Verification items for the finished model (mm, model axes). Face numbers are marked on the shaded views. A direction names the side the tool comes from. Coordinates: 2 decimals unless noted, no trailing zeros. Loops run counter-clockwise (first coordinate to the right, second up) from the corner with the lowest first, then second, coordinate; pieces in that order, holes last.
Q1. Sectioned sample at A-A (x = -2). Enter the section's corners in (y, z), then the cut area to 4 significant figures.
Q2. Sectioned sample at B-B (z = 20). Count the separate pieces of the cut face and the enclosed holes in it, then the cut area to 3 significant figures.
Q3. Mould release check, pull along X, two halves, no side actions. Record for the marked faces 1, 2, 3 and 4: +X half, -X half, draft (parallel to the pull), parting line (faces both ways), or undercut.
Q4. Sectioned sample at C-C (y = -6). Enter the section's corners in (x, z).
Q5. Material ranges on probe 1 along X at (y, z) = (-10, 34); probe 2 along Y at (x, z) = (-66.5, 18); probe 3 along Y at (x, z) = (83, 35), recorded low to high.
Q6. Access from +Z, -Z, +X, -X, +Y, -Y to the whole of each face (thin tool, end or side, straight path). Record for the marked faces 5 and 6.
Q7. Go/stop test with flat-tipped pins: P1, Ø1.2, axis at x = 27.5, z = 39.5, coming from the -Y side; P2, Ø0.8, axis at y = 28, z = 39, coming from the +X side; P3, Ø4, axis at x = 83, y = -35, coming from the +Z side. Record where each tip stops, or that it passes through.
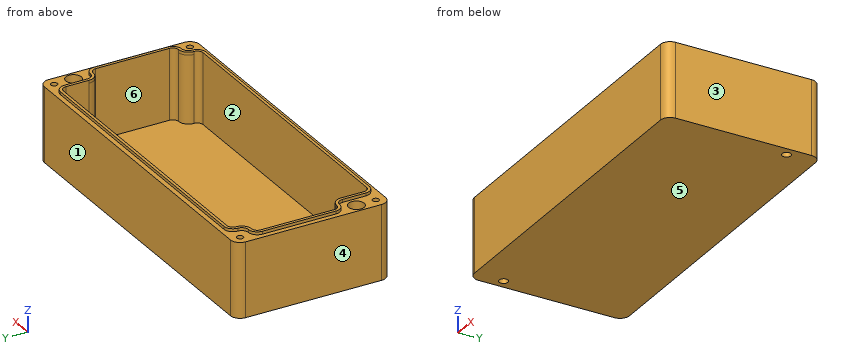
```python
from build123d import *

# Parameters (mm, degrees)
SKETCH1_W                                   = 176
SKETCH1_H                                   = 80
BOSS_EXTRUDE1_DEPTH                         = 38.5
SKETCH2_W                                   = 168
SKETCH2_H                                   = 72
CUT_EXTRUDE1_DEPTH                          = 35
FILLET2_R                                   = 5
SKETCH8_W                                   = 8
SKETCH8_H                                   = 20
SKETCH8_H_2                                 = 8
BOSS_EXTRUDE2_DEPTH                         = 35
FILLET4_R                                   = 3
FILLET5_R                                   = 5
M4_TAPPED_HOLE1_D                           = 3.3
M4_TAPPED_HOLE1_DEPTH                       = 11.5
M4_TAPPED_HOLE1_TIP                         = 0.991420021
BOSS_EXTRUDE3_START                         = 1.5
BOSS_EXTRUDE3_DEPTH                         = 1.5
CBORE_FOR_M4_CHEESE_HEAD_SCREW1_D           = 4.5
CBORE_FOR_M4_CHEESE_HEAD_SCREW1_CBORE_D     = 8
CBORE_FOR_M4_CHEESE_HEAD_SCREW1_CBORE_DEPTH = 30


with BuildPart() as part:
    # Sketch1 → Boss-Extrude1 (new body)
    with BuildSketch(Plane.XY):
        Rectangle(SKETCH1_W, SKETCH1_H)
    extrude(amount=BOSS_EXTRUDE1_DEPTH)

    # Sketch2 → Cut-Extrude1 (cut)
    with BuildSketch(Plane.XY.offset(38.5)):
        Rectangle(SKETCH2_W, SKETCH2_H)
    extrude(amount=-CUT_EXTRUDE1_DEPTH, mode=Mode.SUBTRACT)

    # Fillet2
    fillet2_edges = [part.edges().sort_by_distance(p)[0] for p in [
        (-88, 40, 19.25),
        (88, 40, 19.25),
        (88, -40, 19.25),
        (-88, -40, 19.25),
    ]]
    fillet(fillet2_edges, radius=FILLET2_R)

    # Sketch8 → Boss-Extrude2 (add)
    with BuildSketch(Plane.XY.offset(3.5)):
        with Locations((80, 26)):
            Rectangle(SKETCH8_W, SKETCH8_H)
        with Locations((80, -32)):
            Rectangle(SKETCH8_W, SKETCH8_H_2)
        with Locations((-80, -26)):
            Rectangle(SKETCH8_W, SKETCH8_H)
        with Locations((-80, 32)):
            Rectangle(SKETCH8_W, SKETCH8_H_2)
    extrude(amount=BOSS_EXTRUDE2_DEPTH)

    # Fillet4
    fillet4_edges = [part.edges().sort_by_distance(p)[0] for p in [
        (76, 36, 21),
        (84, 16, 21),
        (84, -28, 21),
        (76, -36, 21),
        (-76, -36, 21),
        (-84, -16, 21),
        (-84, 28, 21),
        (-76, 36, 21),
    ]]
    fillet(fillet4_edges, radius=FILLET4_R)

    # Fillet5
    fillet5_edges = [part.edges().sort_by_distance(p)[0] for p in [
        (-76, -16, 21),
        (76, -28, 21),
        (76, 16, 21),
        (-76, 28, 21),
    ]]
    fillet(fillet5_edges, radius=FILLET5_R - 0.0001)  # a hair under: the kernel refuses the full size

    # M4 Tapped Hole1
    with Locations(Plane.XY.offset(38.5)):
        with Locations((-83, -35), (83, 35), (-83, 35), (83, -35)):
            Hole(M4_TAPPED_HOLE1_D / 2, depth=M4_TAPPED_HOLE1_DEPTH)
            with Locations((0, 0, -(M4_TAPPED_HOLE1_DEPTH + M4_TAPPED_HOLE1_TIP / 2))):  # 118° drill point
                Cone(0, M4_TAPPED_HOLE1_D / 2, M4_TAPPED_HOLE1_TIP, mode=Mode.SUBTRACT)

    # Sketch9 → Boss-Extrude3 (add)
    with BuildSketch(Plane.XY.offset(38.5).offset(BOSS_EXTRUDE3_START)):
        with BuildLine():
            Line((73, 37.5), (-73, 37.5))
            ThreePointArc((-73, 37.5), (-76.181980515, 36.181980515), (-77.5, 33))
            ThreePointArc((-77.5, 33), (-78.525126266, 30.525126266), (-81, 29.5))
            ThreePointArc((-81, 29.5), (-84.181980515, 28.181980515), (-85.5, 25))
            Line((-85.5, 25), (-85.5, -13))
            ThreePointArc((-85.5, -13), (-84.181980515, -16.181980515), (-81, -17.5))
            ThreePointArc((-81, -17.5), (-78.525126266, -18.525126266), (-77.5, -21))
            Line((-77.5, -21), (-77.5, -33))
            ThreePointArc((-77.5, -33), (-76.181980515, -36.181980515), (-73, -37.5))
            Line((-73, -37.5), (73, -37.5))
            ThreePointArc((73, -37.5), (76.181980515, -36.181980515), (77.5, -33))
            ThreePointArc((77.5, -33), (78.525126266, -30.525126266), (81, -29.5))
            ThreePointArc((81, -29.5), (84.181980515, -28.181980515), (85.5, -25))
            Line((85.5, -25), (85.5, 13))
            ThreePointArc((85.5, 13), (84.181980515, 16.181980515), (81, 17.5))
            ThreePointArc((81, 17.5), (78.525126266, 18.525126266), (77.5, 21))
            Line((77.5, 21), (77.5, 33))
            ThreePointArc((77.5, 33), (76.181980515, 36.181980515), (73, 37.5))
        make_face()
        with BuildLine():
            Line((73, 36), (-73, 36))
            ThreePointArc((-73, 36), (-75.121320344, 35.121320344), (-76, 33))
            ThreePointArc((-76, 33), (-77.464466094, 29.464466094), (-81, 28))
            ThreePointArc((-81, 28), (-83.121320344, 27.121320344), (-84, 25))
            Line((-84, 25), (-84, -13))
            ThreePointArc((-84, -13), (-83.121320344, -15.121320344), (-81, -16))
            ThreePointArc((-81, -16), (-77.464466094, -17.464466094), (-76, -21))
            Line((-76, -21), (-76, -33))
            ThreePointArc((-76, -33), (-75.121320344, -35.121320344), (-73, -36))
            Line((-73, -36), (73, -36))
            ThreePointArc((73, -36), (75.121320344, -35.121320344), (76, -33))
            ThreePointArc((76, -33), (77.464466094, -29.464466094), (81, -28))
            ThreePointArc((81, -28), (83.121320344, -27.121320344), (84, -25))
            Line((84, -25), (84, 13))
            ThreePointArc((84, 13), (83.121320344, 15.121320344), (81, 16))
            ThreePointArc((81, 16), (77.464466094, 17.464466094), (76, 21))
            Line((76, 21), (76, 33))
            ThreePointArc((76, 33), (75.121320344, 35.121320344), (73, 36))
        make_face(mode=Mode.SUBTRACT)
    extrude(amount=-BOSS_EXTRUDE3_DEPTH)

    # CBORE for M4 Cheese Head Screw1 (through all)
    with Locations(Plane.XY.offset(38.5)):
        with Locations((83, 25), (-83, -25)):
            CounterBoreHole(CBORE_FOR_M4_CHEESE_HEAD_SCREW1_D / 2, CBORE_FOR_M4_CHEESE_HEAD_SCREW1_CBORE_D / 2, CBORE_FOR_M4_CHEESE_HEAD_SCREW1_CBORE_DEPTH)


solid = part.part
```
Geometry check:
1. outline: (-40, 0) - (40, 0) - (40, 38.5) - (37.5, 38.5) - (37.5, 40) - (36, 40) - (36, 3.5) - (-36, 3.5) - (-36, 40) - (-37.5, 40) - (-37.5, 38.5) - (-40, 38.5) - close
1. area: 564.5 mm2
2. separate pieces: 1
2. enclosed holes: 3
2. area: 2,300 mm2
3. face 1: draft
3. face 2: undercut
3. face 3: +X half
3. face 4: -X half
4. outline: (-88, 0) - (88, 0) - (88, 38.5) - (85.5, 38.5) - (85.5, 40) - (84, 40) - (84, 3.5) - (-84, 3.5) - (-84, 40) - (-85.5, 40) - (-85.5, 38.5) - (-88, 38.5) - close
5. probe 1: x = -88 to -84, 84 to 88
5. probe 2: y = -40 to -36, 36 to 40
5. probe 3: y = -40 to -36.65, -33.35 to -27.24, 15.24 to 21, 29 to 33.35, 36.65 to 40
6. face 5: -Z, +X, -X, +Y, -Y
6. face 6: +Z
7. P1: stops at y = -37.5
7. P2: stops at x = 77.5
7. P3: stops at z = 38.5
